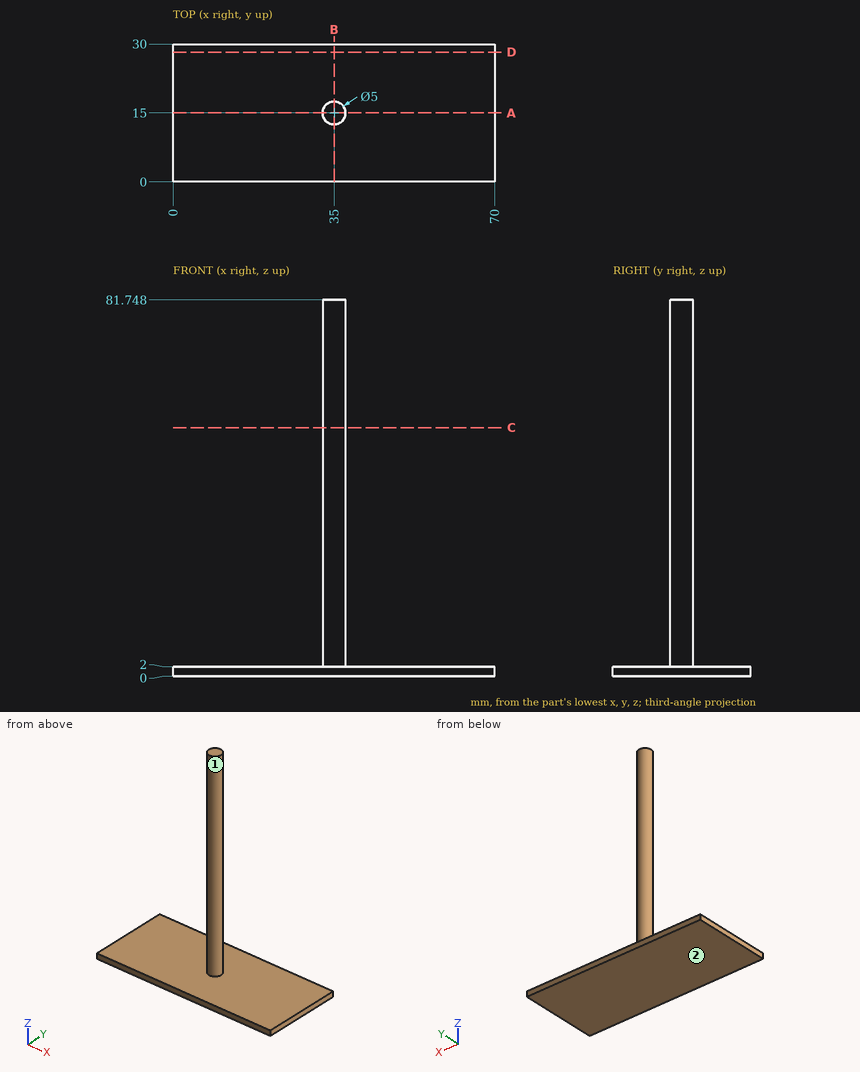
The drawing under review shows one solid part. Ordinate dimensions are in mm from its lowest x, y, z. A direction names the side the tool comes from. Round coordinates to 2 decimals unless told otherwise and drop trailing zeros. Loops run counter-clockwise (first coordinate to the right, second up) from the corner with the lowest first, then second, coordinate; pieces in that order, holes last. Notation, with made-up numbers: (-20, 75.5) -> (19, 75.5) arc R14 cw to (19, 84.5) -> close; hole circle Ø2 at (-15.5, 63.5). An arc over 180 degrees is marked (long way). Answer in a Markdown table with one row per item.
1) Tool access review of the marked faces 1 and 2: name each direction out of +Z, -Z, +X, -X, +Y, -Y from which nothing blocks a thin tool from reaching the whole face with its end or side.
Taken from the geometry:
| item | result |
|---|---|
| face 1 | +Z |
| face 2 | -Z, +X, -X, +Y, -Y |
2) Consider section B-B, the plane x = 35. Write out the cut boundary in (y, z), plus the area to 3 significant figures.
Taken from the geometry:
| item | result |
|---|---|
| outline | (0, 0) -> (30, 0) -> (30, 2) -> (17.5, 2) -> (17.5, 81.75) -> (12.5, 81.75) -> (12.5, 2) -> (0, 2) -> close |
| area | 459 mm² |
3) Consider section C-C, the plane z = 54. Write out the cut boundary in (x, y), plus the area to 3 significant figures.
Taken from the geometry:
| item | result |
|---|---|
| outline | circle Ø5 at (35, 15) |
| area | 19.6 mm² |
4) Consider section D-D, the plane y = 28.25. Write out the cut boundary in (x, z), plus the area to 3 significant figures.
Taken from the geometry:
| item | result |
|---|---|
| outline | (0, 0) -> (70, 0) -> (70, 2) -> (0, 2) -> close |
| area | 140 mm² |
5) For pin 1 Ø8 at (x, y) = (8.5, 7) entering from +Z; pin 2 Ø1 at (x, z) = (39.5, 28.5) entering from +Y, all flat-tipped, find the tip position at first contact; note any pin that passes through.
Taken from the geometry:
| item | result |
|---|---|
| pin 1 | stops at z = 2 |
| pin 2 | passes through |
6) Wall thickness on line 1 along Z through (x, y) = (46.5, 15.75); line 2 along Y through (x, z) = (35, 7.5); line 3 along X through (y, z) = (13.5, 20): over which ranges is each line inside the solid? List them lowest first.
Taken from the geometry:
| item | result |
|---|---|
| line 1 | z = 0 to 2 |
| line 2 | y = 12.5 to 17.5 |
| line 3 | x = 33 to 37 |
7) Consider section A-A, the plane y = 15. Write out the cut boundary in (x, z), plus the area to 3 significant figures.
Taken from the geometry:
| item | result |
|---|---|
| outline | (0, 0) -> (70, 0) -> (70, 2) -> (37.5, 2) -> (37.5, 81.75) -> (32.5, 81.75) -> (32.5, 2) -> (0, 2) -> close |
| area | 539 mm² |
